from build123d import *

# Parameters (mm, degrees)
F2_R     = 0.635
F4_D     = 6.35
F6_D     = 4.445
F7_D     = 2.7051
F7_DEPTH = 20.79725


with BuildPart() as f1:
    # F0 (on Front) → F1 (revolve)
    with BuildSketch(Plane.XZ):
        Polygon((-12.7, 0), (0, 0), (0, 17.145), (-6.35, 17.145), (-8.5497045256, 15.875), (-12.2465454744, 15.875), (-14.44625, 17.145), (-20.79625, 17.145), (-20.79625, 12.8905), (-7.9375, 12.8905), (-7.9375, 6.985), (-12.7, 6.985), align=None)
    revolve(axis=Axis((0, 0, 8.5725), (0, 0, -1)))

    # F2
    f2_edges = [f1.edges().sort_by_distance(p)[0] for p in [
        (12.7, 0, 6.985),
    ]]
    fillet(f2_edges, radius=F2_R)

    # F4 (through all)
    with Locations(Plane.XY.offset(17.145)):
        with Locations((0, 0)):
            Hole(F4_D / 2)

    # F6 (through all)
    with Locations(Plane.XY.offset(17.145)):
        with Locations((-17.62125, 0)):
            Hole(F6_D / 2)

    # F7 (through all, one way)
    with BuildSketch(Plane.XZ):
        with Locations((0, 10)):
            Circle(F7_D / 2)
    extrude(amount=-F7_DEPTH, mode=Mode.SUBTRACT)


solid = f1.part
Check sheet for the modelled part. Datum: model origin and axes. Units: mm. A direction names the side the tool comes from. Round coordinates to 2 decimals unless told otherwise and drop trailing zeros. Loops run counter-clockwise (first coordinate to the right, second up) from the corner with the lowest first, then second, coordinate; pieces in that order, holes last.
1. Sectioned sample at D-D on y = 16.5. Record the boundary of the cut face in (x, z) (1 decimal).
2. Scan lines: probe 1 along Z at (x, y) = (0, -11) (1 decimal); probe 2 along Y at (x, z) = (0, 12) (1 decimal); probe 3 along Z at (x, y) = (12, -11.5) (1 decimal). Record each from-to range of solid material in increasing order.
3. Sectioned sample at C-C on z = 1.75. Record the boundary of the cut face in (x, y) (3 decimals), and give its area (3 significant figures).
4. Set-up check for faces 5 (the cylindrical face through (1.25, 5.37, 9.48)), 6 (the cylindrical face through (2.75, -12.4, 3.13)), 7 (the cylindrical face through (1.72, -7.75, 9.9)), 8 (the flat face through (-8.34, -2.55, 15.875)), 9 (the flat face through (-2, 3, 17.145)): record each of +Z, -Z, +X, -X, +Y, -Y from which the full face is reachable in a straight line by a thin tool's end or side.
5. Mould release check, pull along X, two halves, no side actions. Record for faces 1 (the flat face through (-3, -3, 0)), 2 (the cylindrical face through (2.71, 20.62, 14.99)), 3 (the cylindrical face through (-15.4, 0.1, 15)), 4 (the conical face through (-11.812, 3.72, 15.954)): released by +X, released by -X, zero draft, split by the parting line, or undercut.
6. Sectioned sample at A-A on x = 0. Give the number of separate pieces and of enclosed holes in the cut face, and give its area (3 significant figures).
7. Gauge pin test, flat ends, axial feed: pin 1 Ø6 at (y, z) = (-4, 10.5) entering from -X; pin 2 Ø2 at (x, z) = (-6.5, 2) entering from +Y; pin 3 Ø2 at (x, y) = (0, 14) entering from -Z. Record the tip position at first contact, or that the pin passes through.
Recorded:
1. outline: (-12.7, 12.9) - (12.7, 12.9) - (12.7, 17.1) - (-12.7, 17.1) - close
2. probe 1: z = 0 to 7, 12.9 to 15.9
2. probe 2: y = -7.9 to -3.2, 3.2 to 7.9
2. probe 3: z = 12.9 to 17.1
3. outline: circle Ø25.4 at (0, 0); hole circle Ø6.35 at (0, 0)
3. area: 475 mm2
4. face 5: +Y
4. face 6: -Z
4. face 7: none
4. face 8: +Z
4. face 9: +Z, +X, -X, +Y, -Y
5. face 1: zero draft
5. face 2: split by the parting line
5. face 3: undercut
5. face 4: undercut
6. separate pieces: 3
6. enclosed holes: 0
6. area: 311 mm2
7. pin 1: stops at x = -20.68
7. pin 2: stops at y = 11.45
7. pin 3: stops at z = 12.89
